from build123d import *

# Parameters (mm, degrees)
CUT_EXTRUDE1_DEPTH = 1.8
CIRPATTERN1_COUNT  = 6


with BuildPart() as part:
    # Sketch1 → Revolve1 (revolve)
    with BuildSketch(Plane(origin=(0, 0, 0), x_dir=(0, 0, -1), z_dir=(1, 0, 0)), mode=Mode.PRIVATE) as revolve1_sk:
        with BuildLine():
            Line((-3.5, 0), (-3.5, 2.5))
            ThreePointArc((-3.5, 2.5), (-2.969863274, 3.779863274), (-1.69, 4.31))
            Line((-1.69, 4.31), (0, 4.31))
            Line((0, 4.31), (0, 2.5))
            Line((0, 2.5), (12, 2.5))
            Line((12, 2.5), (12, 0))
            Line((12, 0), (-3.5, 0))
        make_face()
    revolve(revolve1_sk.sketch.rotate(Axis((0, 0, 5.584882278), (0, 0, -1)), 180), axis=Axis((0, 0, 5.584882278), (0, 0, -1)))

    # Sketch2 → Cut-Extrude1 (cut)
    with BuildSketch(Plane.XY.offset(3.5)):
        with BuildLine():
            Line((-0.730783495, 1.265754142), (0, 0))
            Line((0, 0), (0.730783495, 1.265754142))
            ThreePointArc((0.730783495, 1.265754142), (0.512661987, 1.451735511), (0.375261165, 1.703304737))
            ThreePointArc((0.375261165, 1.703304737), (0, 1.975), (-0.375261165, 1.703304737))
            ThreePointArc((-0.375261165, 1.703304737), (-0.512661987, 1.451735511), (-0.730783495, 1.265754142))
        make_face()
    cut_extrude1 = extrude(amount=-CUT_EXTRUDE1_DEPTH, mode=Mode.SUBTRACT)

    # CirPattern1: Cut-Extrude1 ×6 about axis
    cirpattern1_axis = Axis((0, 0, 0), (0, 0, 1))
    for i in range(1, CIRPATTERN1_COUNT):
        add(cut_extrude1.rotate(cirpattern1_axis, i * 360 / CIRPATTERN1_COUNT), mode=Mode.SUBTRACT)


solid = part.part
Build history of the part. All positions in model axes, mm. A direction names the side the tool comes from. Round coordinates to 2 decimals unless told otherwise and drop trailing zeros. Write each loop counter-clockwise with the first axis right and the second up, starting at its lowest first coordinate (ties: lowest second). Pieces come first, ordered by that corner, then holes. Notation, with made-up numbers: (85.5, -38.5) -> (103.5, -38.5) arc R27 cw to (103.5, -12.5) -> close; hole circle Ø1 at (-30.5, -34). An arc over 180 degrees is marked (long way). Use one line per item in the form item = value.
Q1. Band-saw the part on A-A, the plane x = 0. Write the cut outline in (y, z) (3 decimals), then the cut area to 3 significant figures.
Conclusion:
outline = (-4.31, 0) -> (-2.5, 0) -> (-2.5, -12) -> (2.5, -12) -> (2.5, 0) -> (4.31, 0) -> (4.31, 1.69) arc R1.81 ccw to (2.5, 3.5) -> (1.975, 3.5) -> (1.975, 1.7) -> (-1.975, 1.7) -> (-1.975, 3.5) -> (-2.5, 3.5) arc R1.81 ccw to (-4.31, 1.69) -> close
area = 81.7 mm²
Q2. Drop flat-ended pins along their axis: P1, Ø4, axis at x = 3, z = 0, coming from the -Y side; P2, Ø1.5, axis at y = -3, z = -6.5, coming from the -X side; P3, Ø5, axis at y = -0.5, z = -7, coming from the +X side. Give the stop position or say it passes through.
Conclusion:
P1 = -4.19
P2 = -1.09
P3 = 2.5
Q3. Tool access for faces 4 (the cylindrical face through (4.21, 0.93, 0.83)), 5 (the flat face through (2, -2, 0)): list every direction of +Z, -Z, +X, -X, +Y, -Y with a clear straight run to the whole face (end or side of a thin tool).
Conclusion:
face_4 = +Z, -Z
face_5 = -Z
Q4. Band-saw the part on C-C, the plane z = -1. Write the cut outline in (x, y), then the cut area to 3 significant figures.
Conclusion:
outline = circle Ø5 at (0, 0)
area = 19.6 mm²
Q5. Two-plate mould, pull along Y, no slides. Class faces 1 (the flat face through (0, 0, 1.7)), 2 (the cylindrical face through (-0.1, 2.5, -6.1)), 3 (the flat face through (2, 0, 3.5)): released by +Y, released by -Y, zero draft, split by the parting line, or undercut.
Conclusion:
face_1 = undercut
face_2 = split by the parting line
face_3 = zero draft
Q6. Band-saw the part on B-B, the plane z = 2.5. Write the cut outline in (x, y) (3 decimals).
Conclusion:
outline = circle Ø8.237 at (0, 0); hole (-1.663, -0.527) arc R0.395 ccw to (-1.287, -1.177) arc R0.79 cw to (-0.375, -1.703) arc R0.395 ccw to (0.375, -1.703) arc R0.79 cw to (1.287, -1.177) arc R0.395 ccw to (1.663, -0.527) arc R0.79 cw to (1.663, 0.527) arc R0.395 ccw to (1.287, 1.177) arc R0.79 cw to (0.375, 1.703) arc R0.395 ccw to (-0.375, 1.703) arc R0.79 cw to (-1.287, 1.177) arc R0.395 ccw to (-1.663, 0.527) arc R0.79 cw to start
Q7. Drill centre lines: L1, parallel to Y at x = 0.5, z = 2.75; L2, parallel to Z at x = 0, y = 0; L3, parallel to Y at x = 2, z = -9.75. Where is each one in solid material? Low to high.
Conclusion:
L1 = -3.94 to -1.47, 1.47 to 3.94
L2 = -12 to 1.7
L3 = -1.5 to 1.5
